```python
from build123d import *

# Parameters (mm, degrees)
ESQUISSE1_R             = 10
BOSS_EXTRU_1_DEPTH      = 5
ESQUISSE2_R             = 3
ENL_V_MAT_EXTRU_1_DEPTH = 3
ESQUISSE9_R             = 1.5
ENL_V_MAT_EXTRU_2_DEPTH = 3


with BuildPart() as part:
    # Esquisse1 → Boss.-Extru.1 (new body)
    with BuildSketch(Plane.XY):
        Circle(ESQUISSE1_R)
    extrude(amount=BOSS_EXTRU_1_DEPTH)

    # Esquisse2 → Enlèv. mat.-Extru.1 (cut)
    with BuildSketch(Plane.XY.offset(5)):
        Circle(ESQUISSE2_R)
    extrude(amount=-ENL_V_MAT_EXTRU_1_DEPTH, mode=Mode.SUBTRACT)

    # Esquisse3 → Enlèvement de matière-Révolution1 (revolve, cut)
    with BuildSketch(Plane(origin=(0, 0, 0), x_dir=(0, 0, -1), z_dir=(1, 0, 0)), mode=Mode.PRIVATE) as enl_vement_de_mati_re_r_volution1_sk:
        with BuildLine():
            Line((0, 10), (-1, 10))
            ThreePointArc((-1, 10), (-0.292893219, 9.707106781), (0, 9))
            Line((0, 9), (0, 10))
        make_face()
        with BuildLine():
            Line((-4, 10), (-5, 10))
            Line((-5, 10), (-5, 9))
            ThreePointArc((-5, 9), (-4.707106781, 9.707106781), (-4, 10))
        make_face()
    revolve(enl_vement_de_mati_re_r_volution1_sk.sketch.rotate(Axis((0, 0, 5), (0, 0, -1)), 90), axis=Axis((0, 0, 5), (0, 0, -1)), mode=Mode.SUBTRACT)

    # Esquisse9 → Enlèv. mat.-Extru.2 (cut)
    with BuildSketch(Plane(origin=(0, 0, 0), x_dir=(-1, 0, 0), z_dir=(0, 0, -1))):
        Circle(ESQUISSE9_R)
    extrude(amount=-ENL_V_MAT_EXTRU_2_DEPTH, mode=Mode.SUBTRACT)


solid = part.part
```
The model under review builds one solid part; all positions refer to its coordinate system, in mm. A direction names the side the tool comes from. Give positions to 0.01 mm unless a question says otherwise; leave off trailing zeros. Write each loop counter-clockwise with the first axis right and the second up, starting at its lowest first coordinate (ties: lowest second). Pieces come first, ordered by that corner, then holes. Notation, with made-up numbers: (-12.75, -30) -> (34.25, -30) arc R19 cw to (34.25, -20) -> close; hole circle Ø6 at (65.25, 39.5). An arc over 180 degrees is marked (long way). Put each result on its own line as item: value.
(1) The part is to be moulded in two halves that separate along Y. For faces 3 (the cylindrical face through (-2.17, -9.76, 2.48)), 4 (the flat face through (0, -2, 0)), 5 (the cylindrical face through (1.5, 0.07, 0.99)), say which applies: pulls with the +Y half, pulls with the -Y half, needs draft (parallel to the pull), parting line crosses it, or undercut.
Results are:
face 3: parting line crosses it
face 4: needs draft
face 5: undercut
(2) For pin 1 Ø3 at (y, z) = (4.5, 2) entering from +X; pin 2 Ø2 at (y, z) = (-2, 2) entering from +X; pin 3 Ø5 at (x, y) = (0, 0) entering from +Z; pin 4 Ø5 at (x, y) = (-1.5, -0.5) entering from +Z, all flat-tipped, find the tip position at first contact; note any pin that passes through.
Results are:
pin 1: x = 9.54
pin 2: x = 9.95
pin 3: z = 2
pin 4: z = 5
(3) To check wall thickness, follow probe 1 along Y at (x, z) = (0, 1.4); probe 2 along Y at (x, z) = (0, 3); probe 3 along Z at (x, y) = (0, 2.25). State the ranges of each line that lie inside material, in increasing order. Write a range as from..to.
Results are:
probe 1: -10..-1.5, 1.5..10
probe 2: -10..-3, 3..10
probe 3: 0..2
(4) Tool access review of faces 1 (the cylindrical face through (-3, 0, 4)), 2 (the flat face through (0, -4, 5)): name each direction out of +Z, -Z, +X, -X, +Y, -Y from which nothing blocks a thin tool from reaching the whole face with its end or side.
Results are:
face 1: +Z
face 2: +Z, +X, -X, +Y, -Y
(5) We need section A-A, the plane y = 0. Give the boundary of the cut face in (x, z), and give its area (3 significant figures).
Results are:
outline: (-10, 1) arc R1 ccw to (-9, 0) -> (-1.5, 0) -> (-1.5, 2) -> (-3, 2) -> (-3, 5) -> (-9, 5) arc R1 ccw to (-10, 4) -> close; (1.5, 0) -> (9, 0) arc R1 ccw to (10, 1) -> (10, 4) arc R1 ccw to (9, 5) -> (3, 5) -> (3, 2) -> (1.5, 2) -> close
area: 75.1 mm²
